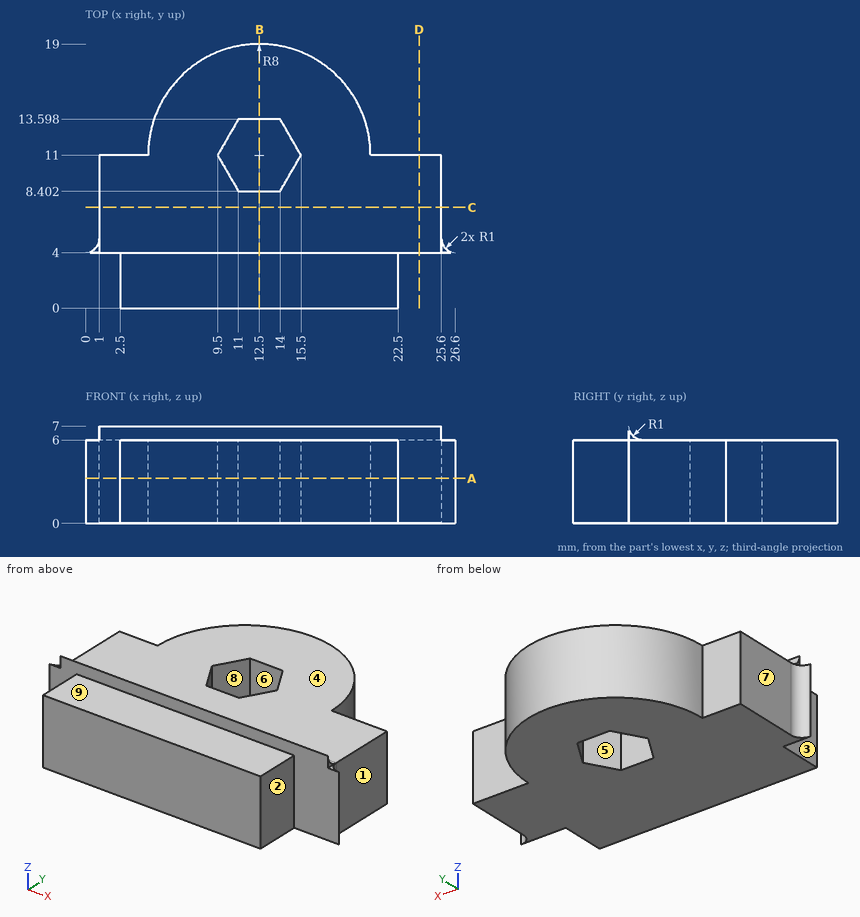
Job drawing, mm, ordinate dimensions from the low corner. One solid piece. A direction names the side the tool comes from. Round coordinates to 2 decimals unless told otherwise and drop trailing zeros. Loops run counter-clockwise (first coordinate to the right, second up) from the corner with the lowest first, then second, coordinate; pieces in that order, holes last.
Item 1: Drop flat-ended pins along their axis: P1, Ø1.8, axis at y = 6.5, z = 4, coming from the -X side; P2, Ø1, axis at y = 2.5, z = 2.5, coming from the +X side; P3, Ø1.8, axis at y = 8.5, z = 3, coming from the +X side. Give the stop position or say it passes through.
Item 2: Drill centre lines: line 1 (Y direction, x = 12.5, z = 1.5); line 2 (Z direction, x = 14, y = 6.5); line 3 (Y direction, x = 24, z = 4.25). Where is each one in solid material? Low to high.
Item 3: Cut at A-A, the plane z = 3.25. Give the cut face in (x, y), then the cut area to 3 significant figures.
Item 4: 3-axis set-ups, long thin cutter, end or side, ignore diameter. For the marked faces 1, 2, 3, 4 and 5: which of +Z, -Z, +X, -X, +Y, -Y reach the whole face in a straight line?
Item 5: Mould opens along X. For the marked faces 6, 7, 8 and 9 say: +X half, -X half, draft (parallel to the pull), parting line (faces both ways), or undercut.
Item 6: Cut at B-B, the plane x = 12.5. Give the cut face in (y, z), then the cut area to 3 significant figures.
Item 7: Cut at C-C, the plane y = 7.25. Give the cut face in (x, z), then the cut area to 3 significant figures.
Item 8: Cut at D-D, the plane x = 24. Give the cut face in (y, z), then the cut area to 3 significant figures.
A:
1. P1: stops at x = 1
1. P2: stops at x = 22.5
1. P3: stops at x = 25.6
2. line 1: y = 0 to 8.4, 13.6 to 19
2. line 2: z = 0 to 6
2. line 3: y = 4 to 11
3. outline: (0, 4) - (2.5, 4) - (2.5, 0) - (22.5, 0) - (22.5, 4) - (26.6, 4) arc R1 cw to (25.6, 5) - (25.6, 11) - (20.5, 11) arc R8 ccw to (4.5, 11) - (1, 11) - (1, 5) arc R1 cw to start; hole (9.5, 11) - (11, 8.4) - (14, 8.4) - (15.5, 11) - (14, 13.6) - (11, 13.6) - close
3. area: 330 mm2
4. face 1: +Z, -Z, +X, +Y
4. face 2: +Z, -Z, +X, -Y
4. face 3: +Z, -Z, -X, -Y
4. face 4: +Z, +X, -X, +Y
4. face 5: +Z, -Z
5. face 6: undercut
5. face 7: -X half
5. face 8: undercut
5. face 9: draft
6. outline: (0, 0) - (8.4, 0) - (8.4, 6) - (5, 6) arc R1 cw to (4, 7) - (4, 6) - (0, 6) - close; (13.6, 0) - (19, 0) - (19, 6) - (13.6, 6) - close
6. area: 83.0 mm2
7. outline: (1, 0) - (25.6, 0) - (25.6, 6) - (1, 6) - close
7. area: 148 mm2
8. outline: (4, 0) - (11, 0) - (11, 6) - (5, 6) arc R1 cw to (4, 7) - close
8. area: 42.2 mm2
